Autodesk Inventor part; units mm, degrees
ref_plane "YZ Plane" through (0, 0, 0) normal (1, 0, 0) x (0, 1, 0)
ref_plane "XZ Plane" through (0, 0, 0) normal (0, 1, 0) x (-1, 0, 0)
ref_plane "XY Plane" through (0, 0, 0) normal (0, 0, 1) x (1, 0, 0)
sketch "スケッチ1" plane through (0, 0, 0) normal (1, 0, 0) x (0, 1, 0)
  line L0 (0, 9.4) -> (0, 0)
  line L1 (0, 0) -> (2.4, 0)
  line L2 (2.4, 0) -> (2.4, 1.4)
  line L3 (2.4, 1.4) -> (1.3, 1.4)
  line L4 (1.3, 1.4) -> (1.3, 9.4)
  line L5 (1.3, 9.4) -> (0, 9.4)
  dimension "d1" = 1.3
  dimension "d2" = 1.4
  dimension "d3" = 2.4
  dimension "d10" = 8
revolve "回転1" add sketch "スケッチ1" angle 360 about axis through (0, 0, 9.4) along (0, 0, -1)
thread "ねじ1"
sketch "スケッチ2" plane through (0, 0, 0) normal (0, 0, -1) x (-1, 0, 0)
  line L0 (0, 0.866) -> (0.75, 0.433)
  line L1 (0.75, 0.433) -> (0.75, -0.433)
  line L2 (0.75, -0.433) -> (0, -0.866)
  line L3 (0, -0.866) -> (-0.75, -0.433)
  line L4 (-0.75, -0.433) -> (-0.75, 0.433)
  line L5 (-0.75, 0.433) -> (0, 0.866)
  circle A0 centre (0, 0) radius 2.4
  line L6 (0, 2.4) -> (0, -2.4) construction
  dimension "d7" = 1.5
extrude "押し出し1" cut sketch "スケッチ2" against normal blind 1.4 contours L0 L1 L2 L3 L4 L5
properties part number "M2_6-8" material "ステンレス鋼 AISI 304"
Source: CAD feature listing. Evaluate the final solid. Frame: model axes, mm. A direction names the side the tool comes from. Give positions to 0.01 mm unless a question says otherwise; leave off trailing zeros. Write each loop counter-clockwise with the first axis right and the second up, starting at its lowest first coordinate (ties: lowest second). Pieces come first, ordered by that corner, then holes. Notation, with made-up numbers: M 24,59 L 63,59 A26 cw 63,88 Z; hole C -5,-24 d10. An arc over 180 degrees is marked long. Return JSON: item names as keys, results as strings. Group by question number.
1) First-contact query: pin 1 Ø1.5 at (y, z) = (0, 6.5) entering from +X; pin 2 Ø2 at (x, z) = (-0.5, 6.5) entering from -Y. Flat tips, straight axial feed; report the tip coordinate or a pass-through.
2) Draft query along Y for faces 4 (the face through (0, 0, 9.4)), 5 (the face through (-1.29, -0.17, 5.46)), 6 (the face through (-0.75, 0, 1)). Return one class per face: released by +Y, released by -Y, zero draft, split by the parting line, or undercut.
3) Set-up query: faces 1 (the face through (-1.03, 1.03, 1.4)), 2 (the face through (0.75, 0, 1)), 3 (the face through (1, -1, 0)). Return all of +Z, -Z, +X, -X, +Y, -Y with unobstructed straight access to the full face (end or side cutting, diameter ignored); none if empty.
4) Cut plane D-D, the plane x = 1.15. Output: boundary loops of the cut face in (y, z).
5) Cut plane C-C, the plane x = 0.4. Output: boundary loops of the cut face in (y, z).
6) Cut plane B-B, the plane y = 0. Output: boundary loops of the cut face in (x, z), then the cut area to 3 significant figures.
7) Ray query, L1, parallel to Z at x = -0.1, y = 0.25; L2, parallel to Z at x = -1.65, y = 0.45; L3, parallel to Y at x = -0.95, z = 7. Return the intervals inside material, ascending.
8) Cut plane A-A, the plane z = 1. Output: boundary loops of the cut face in (x, y).
Data:
{
 "1": {"pin 1": "stops at x = 1.3", "pin 2": "stops at y = -1.3"},
 "2": {"face 4": "zero draft", "face 5": "split by the parting line", "face 6": "undercut"},
 "3": {"face 1": "+Z", "face 2": "-Z", "face 3": "-Z, +X, -X, +Y, -Y"},
 "4": {"outline": "M -2.11,0 L 2.11,0 L 2.11,1.4 L 0.61,1.4 L 0.61,9.4 L -0.61,9.4 L -0.61,1.4 L -2.11,1.4 Z"},
 "5": {"outline": "M -2.37,0 L -0.64,0 L -0.64,1.4 L 0.64,1.4 L 0.64,0 L 2.37,0 L 2.37,1.4 L 1.24,1.4 L 1.24,9.4 L -1.24,9.4 L -1.24,1.4 L -2.37,1.4 Z"},
 "6": {"outline": "M -2.4,0 L -0.75,0 L -0.75,1.4 L 0.75,1.4 L 0.75,0 L 2.4,0 L 2.4,1.4 L 1.3,1.4 L 1.3,9.4 L -1.3,9.4 L -1.3,1.4 L -2.4,1.4 Z", "area": "25.4 mm²"},
 "7": {"L1": "z = 1.4 to 9.4", "L2": "z = 0 to 1.4", "L3": "y = -0.89 to 0.89"},
 "8": {"outline": "C 0,0 d4.8; hole M -0.75,-0.43 L 0,-0.87 L 0.75,-0.43 L 0.75,0.43 L 0,0.87 L -0.75,0.43 Z"}
}
